Verification items for the finished model (mm, model axes). Face numbers are marked on the shaded views. A direction names the side the tool comes from. Round coordinates to 2 decimals unless told otherwise and drop trailing zeros. Order: outer loops, then holes, each group sorted by start corner. A loop starts at its lowest first (then second) coordinate and runs counter-clockwise, first axis right, second up. Notation, with made-up numbers: (-40, -16.75) -> (-3, -16.75) arc R22 ccw to (-3, -9.75) -> close; hole circle Ø8 at (10, 16). An arc over 180 degrees is marked (long way). Put each result on its own line as item: value.
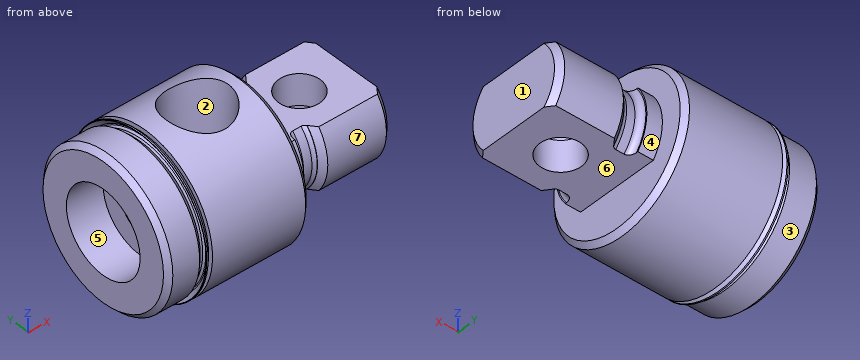
from build123d import *

# Parameters (mm, degrees)
SKETCH3_W               = 47.0408
SKETCH3_H               = 94.0816
SKETCH3_W_2             = 9.4615
SKETCH3_H_2             = 47.0408
CUT_EXTRUDE1_DEPTH      = 15.8877
HOLE1_D                 = 6.35
HOLE1_DEPTH             = 19.08302
HOLE1_TIP               = 1.833087105
SKETCH7_W               = 5.6642
SKETCH7_H               = 6.4135
SKETCH9_R               = 3.2004
CUT_EXTRUDE2_DEPTH      = 7.096125
CUT_EXTRUDE2_DEPTH_BACK = 7.096125


with BuildPart() as part:
    # Sketch1 → Revolve1 (revolve)
    with BuildSketch(Plane.XY):
        Polygon((0, 0), (0, 10.48385), (0.762, 11.24585), (4.8895, 11.24585), (5.6515, 10.48385), (6.4135, 10.48385), (6.4135, 11.7602), (20.7391, 11.7602), (21.5011, 10.9982), (21.5011, 0), align=None)
    revolve(axis=Axis((21.5011, 0, 0), (-1, 0, 0)))

    # Sketch2 → Revolve2 (revolve)
    with BuildSketch(Plane.XY):
        with BuildLine():
            Line((21.5011, 0), (21.5011, 7.90575))
            Line((21.5011, 7.90575), (23.8887, 7.90575))
            Line((23.8887, 7.90575), (23.8887, 7.72795))
            ThreePointArc((23.8887, 7.72795), (24.149082072, 7.099332072), (24.7777, 6.83895))
            Line((24.7777, 6.83895), (26.0604, 6.83895))
            ThreePointArc((26.0604, 6.83895), (26.38140348, 6.898927826), (26.65909292, 7.0707683))
            Line((26.65909292, 7.0707683), (26.689017928, 7.09803))
            Line((26.689017928, 7.09803), (27.528487928, 7.9375))
            Line((27.528487928, 7.9375), (36.54933, 7.9375))
            Line((36.54933, 7.9375), (37.3888, 7.09803))
            Line((37.3888, 7.09803), (37.3888, 0))
            Line((37.3888, 0), (21.5011, 0))
        make_face()
    revolve(axis=Axis((37.3888, 0, 0), (-1, 0, 0)))

    # Sketch3 → Cut-Extrude1 (cut)
    with BuildSketch(Plane(origin=(37.3888, 0, 0), x_dir=(0, 0, -1), z_dir=(1, 0, 0))):
        Rectangle(SKETCH3_W, SKETCH3_H)
        Rectangle(SKETCH3_W_2, SKETCH3_H_2, mode=Mode.SUBTRACT)
    extrude(amount=-CUT_EXTRUDE1_DEPTH, mode=Mode.SUBTRACT)

    # Hole1
    with Locations(Plane.ZY):
        with Locations((0, 0)):
            Hole(HOLE1_D / 2, depth=HOLE1_DEPTH)
            with Locations((0, 0, -(HOLE1_DEPTH + HOLE1_TIP / 2))):  # 120° drill point
                Cone(0, HOLE1_D / 2, HOLE1_TIP, mode=Mode.SUBTRACT)

    # Sketch6 → Cut-Revolve1 (revolve, cut)
    with BuildSketch(Plane(origin=(0, 0, 0), x_dir=(1, 0, 0), z_dir=(0, 0.999847695, 0.017452406))):
        Polygon((14.2748, 0), (18.843078009, 0), (18.843078009, -3.0734), (19.114275925, -11.7602), (14.2748, -11.7602), align=None)
    revolve(axis=Axis((14.2748, -0.20524379, 11.758408865), (0, 0.017452406, -0.999847695)), mode=Mode.SUBTRACT)

    # Sketch7 → Cut-Revolve2 (revolve, cut)
    with BuildSketch(Plane.XY):
        with Locations((2.8321, 3.20675)):
            Rectangle(SKETCH7_W, SKETCH7_H)
    revolve(axis=Axis((5.6642, 0, 0), (-1, 0, 0)), mode=Mode.SUBTRACT)

    # Sketch8 → Revolve3 (revolve)
    with BuildSketch(Plane.XY):
        with BuildLine():
            Line((5.53694893, 11.676031804), (6.291012806, 10.921967928))
            ThreePointArc((6.291012806, 10.921967928), (6.328210245, 10.832165367), (6.291012806, 10.742362806))
            Line((6.291012806, 10.742362806), (6.0325, 10.48385))
            Line((6.0325, 10.48385), (5.6515, 10.48385))
            Line((5.6515, 10.48385), (5.6515, 10.22985))
            Line((5.6515, 10.22985), (6.4135, 10.22985))
            Line((6.4135, 10.22985), (6.4135, 11.08684893))
            Line((6.4135, 11.08684893), (5.74014893, 11.7602))
            Line((5.74014893, 11.7602), (5.53694893, 11.7602))
            Line((5.53694893, 11.7602), (5.53694893, 11.676031804))
        make_face()
    revolve(axis=Axis((6.4135, 0, 0), (-1, 0, 0)))

    # Sketch9 → Cut-Extrude2 (cut, two sides)
    with BuildSketch(Plane.XY) as cut_extrude2_sk:
        with Locations((30.1752, 0)):
            Circle(SKETCH9_R)
    extrude(amount=CUT_EXTRUDE2_DEPTH, mode=Mode.SUBTRACT)
    extrude(cut_extrude2_sk.sketch, amount=-CUT_EXTRUDE2_DEPTH_BACK, mode=Mode.SUBTRACT)


solid = part.part
Item 1: Release check for a two-part mould opening along X. For the marked faces 1, 2 and 3 record: +X half, -X half, draft (parallel to the pull), parting line (faces both ways), or undercut.
Check sheet entries:
face 1: +X half
face 2: undercut
face 3: draft
Item 2: Section check A-A on x = 22. Record the boundary of the cut face in (y, z).
Check sheet entries:
outline: (-6.33, -4.73) -> (6.33, -4.73) arc R7.91 ccw to (6.33, 4.73) -> (-6.33, 4.73) arc R7.91 ccw to start
Item 3: Gauge pin test, flat ends, axial feed: pin 1 Ø12 at (x, z) = (23, -7.5) entering from -Y; pin 2 Ø1.5 at (x, y) = (13.5, 1.5) entering from -Z; pin 3 Ø14 at (x, y) = (29, 0) entering from +Z. Record the tip position at first contact, or that the pin passes through.
Check sheet entries:
pin 1: stops at y = -11.6
pin 2: stops at z = -11.74
pin 3: stops at z = 4.73
Item 4: Material ranges on L1, parallel to Y at x = 4.25, z = 0; L2, parallel to X at y = -9, z = 3; L3, parallel to Z at x = 36.5, y = -2.75, recorded low to high. Write a range as [from, to].
Check sheet entries:
L1: y = [-11.25, -6.41], [6.41, 11.25]
L2: x = [0, 21.5]
L3: z = [-4.73, 4.73]
Item 5: Tool access check on the marked faces 4, 5, 6 and 7. Record the directions out of +Z, -Z, +X, -X, +Y, -Y that give a thin tool (end or side, any length) a straight path to the whole face; none if there is none.
Check sheet entries:
face 4: +Y
face 5: -X
face 6: -Z, +X, +Y, -Y
face 7: +X, -Y
Item 6: Section check B-B on y = 1.5. State how many separate pieces and enclosed holes the cut face has, then the cut area to 3 significant figures.
Check sheet entries:
separate pieces: 3
enclosed holes: 0
area: 362 mm^2
